```python
from build123d import *

# Parameters (mm, degrees)
SKETCH1_W           = 292.1
SKETCH1_H           = 89.8
SKETCH1_R           = 14.2875
SKETCH1_R_2         = 2.54
SKETCH1_R_3         = 17.145
BOSS_EXTRUDE1_DEPTH = 6.35
SKETCH2_R           = 2.05
CUT_EXTRUDE1_DEPTH  = 10
SKETCH3_R           = 1.55
SKETCH3_R_2         = 2.05
SKETCH3_R_3         = 1.5
CUT_EXTRUDE2_DEPTH  = 10
FILLET1_R           = 2
SKETCH4_R           = 2.05
SKETCH4_R_2         = 1.778
CUT_EXTRUDE4_DEPTH  = 7.35
SCALE1_SCALE        = 0.333333333


with BuildPart() as part:
    # Sketch1 → Boss-Extrude1 (new body)
    with BuildSketch(Plane.XY):
        with Locations((146.05, 44.9)):
            Rectangle(SKETCH1_W, SKETCH1_H)
        with Locations((146.05, 44.9)):
            Circle(SKETCH1_R, mode=Mode.SUBTRACT)
        with Locations((103.051585406, 62.859439014)):
            Circle(SKETCH1_R_2, mode=Mode.SUBTRACT)
        with Locations((103.049439014, 26.938414594)):
            Circle(SKETCH1_R_2, mode=Mode.SUBTRACT)
        with Locations((67.128414594, 26.940560986)):
            Circle(SKETCH1_R_2, mode=Mode.SUBTRACT)
        with Locations((67.130560986, 62.861585406)):
            Circle(SKETCH1_R_2, mode=Mode.SUBTRACT)
        with Locations((85.09, 44.9)):
            Circle(SKETCH1_R_3, mode=Mode.SUBTRACT)
        with Locations((189.050560986, 62.861585406)):
            Circle(SKETCH1_R_2, mode=Mode.SUBTRACT)
        with Locations((224.971585406, 62.859439014)):
            Circle(SKETCH1_R_2, mode=Mode.SUBTRACT)
        with Locations((224.969439014, 26.938414594)):
            Circle(SKETCH1_R_2, mode=Mode.SUBTRACT)
        with Locations((189.048414594, 26.940560986)):
            Circle(SKETCH1_R_2, mode=Mode.SUBTRACT)
        with Locations((207.01, 44.9)):
            Circle(SKETCH1_R_3, mode=Mode.SUBTRACT)
    extrude(amount=BOSS_EXTRUDE1_DEPTH)

    # Sketch2 → Cut-Extrude1 (cut)
    with BuildSketch(Plane.XY.offset(6.35)):
        with Locations((118.55, 20)):
            Circle(SKETCH2_R)
        with Locations((118.55, 69.8)):
            Circle(SKETCH2_R)
        with Locations((173.55, 20)):
            Circle(SKETCH2_R)
        with Locations((173.55, 69.8)):
            Circle(SKETCH2_R)
    extrude(amount=-CUT_EXTRUDE1_DEPTH, mode=Mode.SUBTRACT)

    # Sketch3 → Cut-Extrude2 (cut)
    with BuildSketch(Plane.XY.offset(6.35)):
        with Locations((284.6, 7.5)):
            Circle(SKETCH3_R)
        with Locations((7.5, 7.5)):
            Circle(SKETCH3_R)
        with Locations((7.5, 82.3)):
            Circle(SKETCH3_R)
        with Locations((284.6, 82.3)):
            Circle(SKETCH3_R)
        with Locations((274.6, 20)):
            Circle(SKETCH3_R_2)
        with Locations((17.5, 20)):
            Circle(SKETCH3_R_2)
        with Locations((17.5, 69.8)):
            Circle(SKETCH3_R_2)
        with Locations((274.6, 69.8)):
            Circle(SKETCH3_R_2)
        with Locations((173.55, 7.5)):
            Circle(SKETCH3_R_3)
        with Locations((173.55, 82.3)):
            Circle(SKETCH3_R_3)
        with Locations((118.55, 82.3)):
            Circle(SKETCH3_R_3)
        with Locations((118.55, 7.5)):
            Circle(SKETCH3_R_3)
    extrude(amount=-CUT_EXTRUDE2_DEPTH, mode=Mode.SUBTRACT)

    # Fillet1
    fillet1_edges = [part.edges().sort_by_distance(p)[0] for p in [
        (0, 89.8, 3.175),
        (292.1, 89.8, 3.175),
        (292.1, 0, 3.175),
        (0, 0, 3.175),
    ]]
    fillet(fillet1_edges, radius=FILLET1_R)

    # Sketch4 → Cut-Extrude4 (cut, through all)
    with BuildSketch(Plane.XY.offset(6.35)):
        with Locations((233.55, 20)):
            Circle(SKETCH4_R)
        with Locations((233.55, 69.8)):
            Circle(SKETCH4_R_2)
        with Locations((58.55, 69.8)):
            Circle(SKETCH4_R_2)
        with Locations((58.55, 20)):
            Circle(SKETCH4_R_2)
    extrude(amount=-CUT_EXTRUDE4_DEPTH, mode=Mode.SUBTRACT)


with BuildPart() as part_1:
    # Scale1: scaled about (146.037752534, 44.903485279, 3.175)
    add(part.part.scale(SCALE1_SCALE).moved(Location((97.358501689, 29.935656853, 2.116666667))))


solid = part_1.part
```
Model file for the job. Use its own axes, mm. Round coordinates to 2 decimals unless told otherwise and drop trailing zeros. Write each loop counter-clockwise with the first axis right and the second up, starting at its lowest first coordinate (ties: lowest second). Pieces come first, ordered by that corner, then holes. Notation, with made-up numbers: (66, -1.5) - (109, -1.5) arc R22 cw to (109, 30.5) - close; hole circle Ø5 at (87, 70.25). An arc over 180 degrees is marked (long way). Use CSV: the item, a comma, the result in double quotes. Start each with the question number.
Item 1: Band-saw the part on A-A (y = 46.5). Write the cut outline in (x, z).
Item 2: Band-saw the part on C-C (z = 3.8). State how many separate pieces and enclosed holes the cut face has, and give its area (3 significant figures).
Item 3: Drill centre lines: L1, parallel to X at y = 38.75, z = 2.8; L2, parallel to Y at x = 172.5, z = 3.45; L3, parallel to X at y = 49.25, z = 3.6. Where is each one in solid material? Low to high. Write a range as [from, to].
Item 4: Band-saw the part on B-B (x = 122). Write the cut outline in (y, z).
Item 5: Two-plate mould, pull along Y, no slides. Class faces 1 (the face through (145, 52, 2.117)), 2 (the face through (145, 29.936, 3)), 3 (the face through (165.62, 50.57, 3.16)): released by +Y, released by -Y, zero draft, split by the parting line, or undercut.
Checked values:
1,outline,"(97.36, 2.12) - (120.23, 2.12) - (120.23, 4.23) - (97.36, 4.23) - close; (131.21, 2.12) - (141.56, 2.12) - (141.56, 4.23) - (131.21, 4.23) - close; (150.53, 2.12) - (160.87, 2.12) - (160.87, 4.23) - (150.53, 4.23) - close; (171.85, 2.12) - (194.73, 2.12) - (194.73, 4.23) - (171.85, 4.23) - close"
2,separate pieces,"1"
2,enclosed holes,"31"
2,area,"2,600 mm²"
3,L1,"x = [97.36, 118.9], [120.56, 130.88], [132.54, 159.54], [161.2, 171.52], [173.18, 194.73]"
3,L2,"y = [29.94, 38.08], [39.75, 50.06], [51.72, 59.87]"
3,L3,"x = [97.36, 122.01], [129.43, 144.1], [147.99, 162.65], [170.07, 194.73]"
4,outline,"(29.94, 2.12) - (40.57, 2.12) - (40.57, 4.23) - (29.94, 4.23) - close; (49.24, 2.12) - (59.87, 2.12) - (59.87, 4.23) - (49.24, 4.23) - close"
5,face 1,"zero draft"
5,face 2,"released by -Y"
5,face 3,"undercut"
